Here's how the part is built. I have some questions about the finished solid (model axes, mm). A direction names the side the tool comes from. Coordinates: 2 decimals unless noted, no trailing zeros. Order: outer loops, then holes, each group sorted by start corner. A loop starts at its lowest first (then second) coordinate and runs counter-clockwise, first axis right, second up.
```python
from build123d import *

# Parameters (mm, degrees)
F1_DEPTH  = 68
F2_R      = 3.8
F3_R      = 6.8
F4_R      = 5
F5_R      = 5.1
F5_R_2    = 3.5
F6_DEPTH  = 120.001
F7_R      = 5.1
F7_R_2    = 3.5
F8_DEPTH  = 120.001
F9_R      = 8.5
F10_DEPTH = 1.5
F11_R     = 8.5
F12_DEPTH = 1.5


with BuildPart() as f1:
    # F0 (on Front) → F1 (new body)
    with BuildSketch(Plane.XZ):
        Polygon((3, 120), (0, 120), (0, 0), (120, 0), (120, 3), (3, 3), align=None)
    extrude(amount=-F1_DEPTH)

    # F2
    f2_edges = [f1.edges().sort_by_distance(p)[0] for p in [
        (3, 34, 3),
    ]]
    fillet(f2_edges, radius=F2_R)

    # F3
    f3_edges = [f1.edges().sort_by_distance(p)[0] for p in [
        (0, 34, 0),
    ]]
    fillet(f3_edges, radius=F3_R)

    # F4
    f4_edges = [f1.edges().sort_by_distance(p)[0] for p in [
        (1.5, 0, 120),
        (120, 0, 1.5),
        (120, 68, 1.5),
        (1.5, 68, 120),
    ]]
    fillet(f4_edges, radius=F4_R)

    # F5 (on face) → F6 (cut, through all)
    with BuildSketch(Plane(origin=(0, 0, 0), x_dir=(1, 0, 0), z_dir=(0, 0, -1))):
        with Locations((108, -34)):
            Circle(F5_R)
        with Locations((38, -34)):
            Circle(F5_R)
        with Locations((58, -14)):
            Circle(F5_R_2)
        with Locations((58, -54)):
            Circle(F5_R_2)
    extrude(amount=-F6_DEPTH, mode=Mode.SUBTRACT)

    # F7 (on face) → F8 (cut, through all)
    with BuildSketch(Plane(origin=(0, 0, 0), x_dir=(0, -1, 0), z_dir=(-1, 0, 0))):
        with Locations((-34, 108)):
            Circle(F7_R)
        with Locations((-34, 38)):
            Circle(F7_R)
        with Locations((-14, 58)):
            Circle(F7_R_2)
        with Locations((-54, 58)):
            Circle(F7_R_2)
    extrude(amount=-F8_DEPTH, mode=Mode.SUBTRACT)

    # F9 (on face) → F10 (cut)
    with BuildSketch(Plane(origin=(0, 0, 0), x_dir=(0, -1, 0), z_dir=(-1, 0, 0))):
        with Locations((-34, 108)):
            Circle(F9_R)
        with Locations((-34, 38)):
            Circle(F9_R)
    extrude(amount=-F10_DEPTH, mode=Mode.SUBTRACT)

    # F11 (on face) → F12 (cut)
    with BuildSketch(Plane(origin=(0, 0, 0), x_dir=(1, 0, 0), z_dir=(0, 0, -1))):
        with Locations((38, -34)):
            Circle(F11_R)
        with Locations((108, -34)):
            Circle(F11_R)
    extrude(amount=-F12_DEPTH, mode=Mode.SUBTRACT)


solid = f1.part
```
Q1. If we section it at C-C on y = 14: Write out the boundary of the cut face in (x, z), then the cut area to 3 significant figures.
Q2. If we section it at A-A on z = 58: Write out the boundary of the cut face in (x, y), then the cut area to 3 significant figures.
Q3. I need wall thicknesses on L1, parallel to Y at x = 58, z = 0.7; L2, parallel to X at y = 64.5, z = 49. Which ranges of each line are inside material? Lowest first, please.
Q4. Will these pins go through, and if not, where does the flat tip stop? pin 1 (1.5 mm diameter, centred on y = 42, z = 51.5, fed in from +X); pin 2 (6.5 mm diameter, centred on y = 54, z = 58, fed in from -X); pin 3 (11.5 mm diameter, centred on x = 108, y = 34, fed in from +Z); pin 4 (16.5 mm diameter, centred on y = 34, z = 108, fed in from -X).
Q5. If we section it at B-B on x = 108: Write out the boundary of the cut face in (y, z).
Q6. For faces 1 (the cylindrical face through (0.74, 30.08, 100.46)), 2 (the cylindrical face through (106.16, 42.3, 0.74)), 3 (the flat face through (2, 34, 120)), which set-ups out of +Z, -Z, +X, -X, +Y, -Y let a thin tool reach every point of the face, with its end or its side?
Q7. We'd pull the mould along Z, two halves only. Please class faces 4 (the flat face through (42, 38, 1.5)), 5 (the flat face through (64, 34, 3)), 6 (the cylindrical face through (1.479, 57.497, 58.154)): pulls with the +Z half, pulls with the -Z half, needs draft (parallel to the pull), parting line crosses it, or undercut.
Q8. If we section it at D-D on z = 108: Write out the boundary of the cut face in (x, y).
Reply:
1. outline: (0, 6.8) arc R6.8 ccw to (6.8, 0) - (54.5, 0) - (54.5, 3) - (6.8, 3) arc R3.8 cw to (3, 6.8) - (3, 54.5) - (0, 54.5) - close; (0, 61.5) - (3, 61.5) - (3, 120) - (0, 120) - close; (61.5, 0) - (120, 0) - (120, 3) - (61.5, 3) - close
1. area: 662 mm2
2. outline: (0, 0) - (3, 0) - (3, 10.5) - (0, 10.5) - close; (0, 17.5) - (3, 17.5) - (3, 50.5) - (0, 50.5) - close; (0, 57.5) - (3, 57.5) - (3, 68) - (0, 68) - close
2. area: 162 mm2
3. L1: y = 0 to 10.5, 17.5 to 50.5, 57.5 to 68
3. L2: x = 0 to 3
4. pin 1: stops at x = 3
4. pin 2: passes through
4. pin 3: stops at z = 3
4. pin 4: stops at x = 1.5
5. outline: (0, 0) - (25.5, 0) - (25.5, 1.5) - (28.9, 1.5) - (28.9, 3) - (0, 3) - close; (39.1, 1.5) - (42.5, 1.5) - (42.5, 0) - (68, 0) - (68, 3) - (39.1, 3) - close
6. face 1: -X
6. face 2: -Z
6. face 3: +Z, +X, -X, +Y, -Y
7. face 4: pulls with the -Z half
7. face 5: pulls with the +Z half
7. face 6: undercut
8. outline: (0, 0) - (3, 0) - (3, 28.9) - (1.5, 28.9) - (1.5, 25.5) - (0, 25.5) - close; (0, 42.5) - (1.5, 42.5) - (1.5, 39.1) - (3, 39.1) - (3, 68) - (0, 68) - close
